from build123d import *

# Parameters (mm, degrees)
SKETCH1_R           = 2.95
BOSS_EXTRUDE1_DEPTH = 6
BOSS_EXTRUDE2_DEPTH = 26.3
BOSS_EXTRUDE3_DEPTH = 6
SKETCH5_R           = 2.95
SKETCH5_R_2         = 1.7
BOSS_EXTRUDE4_DEPTH = 3


with BuildPart() as part:
    # Sketch1 → Boss-Extrude1 (new body)
    with BuildSketch(Plane.XY):
        with BuildLine():
            Line((0, 0), (20, 0))
            Line((20, 0), (20, 4))
            Line((20, 4), (23.6, 4))
            Line((23.6, 4), (23.6, 11))
            Line((23.6, 11), (17.3, 11))
            ThreePointArc((17.3, 11), (9.3, 19), (1.3, 11))
            Line((1.3, 11), (-2.7, 11))
            Line((-2.7, 11), (-2.7, 4))
            Line((-2.7, 4), (0, 4))
            Line((0, 4), (0, 0))
        make_face()
        with Locations((9.3, 11)):
            Circle(SKETCH1_R, mode=Mode.SUBTRACT)
    extrude(amount=BOSS_EXTRUDE1_DEPTH)

    # Sketch2 → Boss-Extrude2 (add)
    with BuildSketch(Plane.ZY.offset(2.7)):
        with BuildLine():
            Line((6, 4), (6, 5))
            ThreePointArc((6, 5), (6.292893219, 4.292893219), (7, 4))
            Line((7, 4), (6, 4))
        make_face()
        with BuildLine():
            Line((0, 4), (-1, 4))
            ThreePointArc((-1, 4), (-0.292893219, 4.292893219), (0, 5))
            Line((0, 5), (0, 4))
        make_face()
    extrude(amount=-BOSS_EXTRUDE2_DEPTH)

    # Sketch4 → Boss-Extrude3 (add)
    with BuildSketch(Plane.XY.offset(6)):
        with BuildLine():
            Line((23.1, 4), (23.1, 5))
            ThreePointArc((23.1, 5), (23.392893219, 4.292893219), (24.1, 4))
            Line((24.1, 4), (23.1, 4))
        make_face()
        with BuildLine():
            Line((-1.5, 4), (-2.5, 4))
            ThreePointArc((-2.5, 4), (-1.792893219, 4.292893219), (-1.5, 5))
            Line((-1.5, 5), (-1.5, 4))
        make_face()
    extrude(amount=-BOSS_EXTRUDE3_DEPTH)

    # Sketch5 → Boss-Extrude4 (add)
    with BuildSketch(Plane(origin=(0, 0, 0), x_dir=(-1, 0, 0), z_dir=(0, 0, -1))):
        with Locations((-9.3, 11)):
            Circle(SKETCH5_R)
        with Locations((-9.3, 11)):
            Circle(SKETCH5_R_2, mode=Mode.SUBTRACT)
    extrude(amount=-BOSS_EXTRUDE4_DEPTH)


solid = part.part
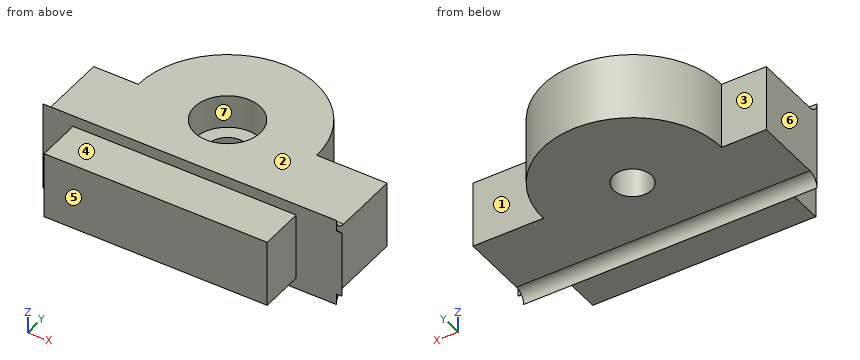
Model file for the job. Use its own axes, mm. Face numbers are marked on the shaded views. A direction names the side the tool comes from. Give positions to 0.01 mm unless a question says otherwise; leave off trailing zeros. Loops run counter-clockwise (first coordinate to the right, second up) from the corner with the lowest first, then second, coordinate; pieces in that order, holes last.
Item 1: Slice it at D-D (x = 0.75). Write the cut outline in (y, z), plus the area to 3 significant figures.
Check values:
outline: (0, 0) - (4, 0) - (4, -1) arc R1 cw to (5, 0) - (11, 0) - (11, 6) - (5, 6) arc R1 cw to (4, 7) - (4, 6) - (0, 6) - close
area: 66.4 mm2
Item 2: Slice it at A-A (x = 9.3). Write the cut outline in (y, z), plus the area to 3 significant figures.
Check values:
outline: (0, 0) - (4, 0) - (4, -1) arc R1 cw to (5, 0) - (9.3, 0) - (9.3, 3) - (8.05, 3) - (8.05, 6) - (5, 6) arc R1 cw to (4, 7) - (4, 6) - (0, 6) - close; (12.7, 0) - (19, 0) - (19, 6) - (13.95, 6) - (13.95, 3) - (12.7, 3) - close
area: 86.5 mm2
Item 3: Drop flat-ended pins along their axis: P1, Ø7.5, axis at x = 9.3, y = 11, coming from the +Z side; P2, Ø1, axis at y = 2.5, z = 6, coming from the +X side; P3, Ø4, axis at y = 7, z = 4, coming from the +X side; P4, Ø2.5, axis at x = 9.3, y = 11, coming from the +Z side. Give the stop position or say it passes through.
Check values:
P1: stops at z = 6
P2: stops at x = 20
P3: stops at x = 23.6
P4: passes through
Item 4: Mould opens along X. For the marked faces 5, 6 and 7 say: +X half, -X half, draft (parallel to the pull), parting line (faces both ways), or undercut.
Check values:
face 5: draft
face 6: -X half
face 7: undercut
Item 5: Slice it at B-B (z = 5.5). Write the cut outline in (x, y).
Check values:
outline: (-2.7, 4) - (0, 4) - (0, 0) - (20, 0) - (20, 4) - (24.1, 4) arc R1 cw to (23.6, 4.13) - (23.6, 11) - (17.3, 11) arc R8 ccw to (1.3, 11) - (-2.7, 11) - close; hole circle Ø5.9 at (9.3, 11)
Item 6: Slice it at C-C (y = 13.5). Write the cut outline in (x, z).
Check values:
outline: (1.7, 0) - (16.9, 0) - (16.9, 6) - (10.87, 6) - (10.87, 3) - (7.73, 3) - (7.73, 6) - (1.7, 6) - close
Item 7: Drill centre lines: line 1 along Y through (x, z) = (9.3, 1.6); line 2 along Y through (x, z) = (9.3, 3.85); line 3 along X through (y, z) = (10.75, 1.5). Where is each one in solid material? Low to high.
Check values:
line 1: y = 0 to 9.3, 12.7 to 19
line 2: y = 0 to 8.05, 13.95 to 19
line 3: x = -2.7 to 7.62, 10.98 to 23.6
Item 8: Which spindle directions (+Z, -Z, +X, -X, +Y, -Y) get a long thin tool onto all of the face, cutting with end or side? Do the marked faces 1, 2, 3 and 4. Say none if no direction does.
Check values:
face 1: +Z, -Z, +X, +Y
face 2: +Z, +X, -X, +Y
face 3: +Z, -Z, -X, +Y
face 4: +Z, +X, -X, -Y
